from build123d import *

# Parameters (mm, degrees)
BOSS_EXTRUDE1_DEPTH = 19
HOLE1_D             = 6.75
HOLE1_DEPTH         = 100
HOLE1_CBORE_D       = 23.785
HOLE1_CBORE_DEPTH   = 5


with BuildPart() as part:
    # Sketch1 → Boss-Extrude1 (new body)
    with BuildSketch(Plane.XY):
        with BuildLine():
            Line((12.7, 0), (25.4, 0))
            Line((25.4, 0), (25.4, 19))
            Line((25.4, 19), (-25.4, 19))
            Line((-25.4, 19), (-25.4, 0))
            Line((-25.4, 0), (-12.7, 0))
            ThreePointArc((-12.7, 0), (0, 12.7), (12.7, 0))
        make_face()
    extrude(amount=BOSS_EXTRUDE1_DEPTH)

    # Hole1
    with Locations(Plane(origin=(0, 19, 0), x_dir=(1, 0, 0), z_dir=(0, 1, 0))):
        with Locations((19.05, -9.5), (-19.05, -9.5)):
            CounterBoreHole(HOLE1_D / 2, HOLE1_CBORE_D / 2, HOLE1_CBORE_DEPTH, depth=HOLE1_DEPTH)


solid = part.part
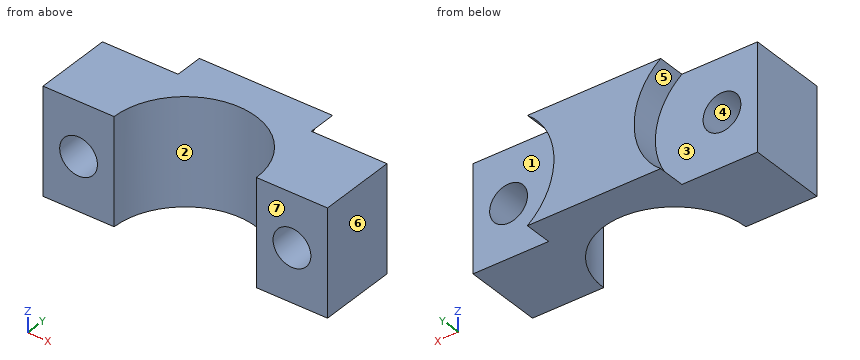
Design review of the part built by this model. Coordinates are the model's own, in mm. Face numbers are marked on the shaded views. A direction names the side the tool comes from. Give positions to 0.01 mm unless a question says otherwise; leave off trailing zeros. Write each loop counter-clockwise with the first axis right and the second up, starting at its lowest first coordinate (ties: lowest second). Pieces come first, ordered by that corner, then holes. Notation, with made-up numbers: M -33,56.5 L 6,56.5 A13 ccw 6,64.5 Z; hole C -31,41.5 d4. An arc over 180 degrees is marked long. Return JSON: item names as keys, results as strings. Group by question number.
Item 1: Tool access review of the marked faces 1, 2 and 3: name each direction out of +Z, -Z, +X, -X, +Y, -Y from which nothing blocks a thin tool from reaching the whole face with its end or side.
Item 2: Take a section at A-A (y = 3). Give the boundary of the cut face in (x, z) (3 decimals).
Item 3: Take a section at D-D (y = 10). Give the boundary of the cut face in (x, z) (3 decimals), plus the area to 3 significant figures.
Item 4: Take a section at B-B (z = 9.5). Give the boundary of the cut face in (x, y) (1 decimal).
Item 5: Clearance check with flat-ended pins moving along their axes: pin 1 Ø5.5 at (x, z) = (-12.5, 10.5) entering from +Y; pin 2 Ø6 at (x, z) = (-19.05, 9.5) entering from +Y; pin 3 Ø1.5 at (y, z) = (16, 4.5) entering from +X. State where each tip first meets the part, or that it passes through.
Item 6: Wall thickness on line 1 along X through (y, z) = (6.25, 9.5) (3 decimals); line 2 along Z through (x, y) = (19.05, 8.5) (3 decimals); line 3 along X through (y, z) = (9.5, 9.5) (3 decimals): over which ranges is each line inside the solid? List them lowest first.
Item 7: The part is to be moulded in two halves that separate along X. For the marked faces 4, 5, 6 and 7, say which applies: pulls with the +X half, pulls with the -X half, needs draft (parallel to the pull), parting line crosses it, or undercut.
Item 8: Take a section at C-C (x = 19.05). Give the boundary of the cut face in (y, z) (3 decimals), plus the area to 4 significant figures.
Return value:
{
 "1": {"face 1": "+X, +Y", "face 2": "+Z, -Z, -Y", "face 3": "-X, +Y"},
 "2": {"outline": "M -25.4,0 L -12.341,0 L -12.341,19 L -25.4,19 Z; M 12.341,0 L 25.4,0 L 25.4,19 L 12.341,19 Z; hole C -19.05,9.5 d6.75; hole C 19.05,9.5 d6.75"},
 "3": {"outline": "M -25.4,0 L -7.829,0 L -7.829,19 L -25.4,19 Z; M 7.829,0 L 25.4,0 L 25.4,19 L 7.829,19 Z; hole C -19.05,9.5 d6.75; hole C 19.05,9.5 d6.75", "area": "596 mm2"},
 "4": {"outline": "M -25.4,0 L -22.4,0 L -22.4,14 L -25.4,14 Z; M -15.7,0 L -12.7,0 A12.7 cw 12.7,0 L 15.7,0 L 15.7,14 L 7.2,14 L 7.2,19 L -7.2,19 L -7.2,14 L -15.7,14 Z; M 22.4,0 L 25.4,0 L 25.4,14 L 22.4,14 Z"},
 "5": {"pin 1": "stops at y = 14", "pin 2": "passes through", "pin 3": "stops at x = 8.64"},
 "6": {"line 1": "x = -25.4 to -22.425, -15.675 to -11.056, 11.056 to 15.675, 22.425 to 25.4", "line 2": "z = 0 to 6.125, 12.875 to 19", "line 3": "x = -25.4 to -22.425, -15.675 to -8.429, 8.429 to 15.675, 22.425 to 25.4"},
 "7": {"face 4": "undercut", "face 5": "pulls with the -X half", "face 6": "pulls with the +X half", "face 7": "needs draft"},
 "8": {"outline": "M 0,0 L 14,0 L 14,6.125 L 0,6.125 Z; M 0,12.875 L 14,12.875 L 14,19 L 0,19 Z", "area": "171.5 mm2"}
}
